Part print with two shaded views. Sizes in mm from the minimum x, y, z corner. A direction names the side the tool comes from. Give positions to 0.01 mm unless a question says otherwise; leave off trailing zeros. Write each loop counter-clockwise with the first axis right and the second up, starting at its lowest first coordinate (ties: lowest second). Pieces come first, ordered by that corner, then holes. Notation, with made-up numbers: (22, -18.5) -> (28, -18.5) arc R14 ccw to (28, -1.5) -> close; hole circle Ø3 at (-35, 38.5). An arc over 180 degrees is marked (long way). Write item = value, one per line. Start each with the question number.
Q1. Saw through at A-A, the plane y = 37.5. List the corners of the cut face in (x, z).
Q2. Mould opens along X. For the marked faces 1, 2, 3 and 4 say: pulls with the +X half, pulls with the -X half, needs draft (parallel to the pull), parting line crosses it, or undercut.
Q3. Saw through at D-D, the plane x = 33. List the corners of the cut face in (y, z).
Q4. Tool access for the marked faces 5, 6 and 7: list every direction of +Z, -Z, +X, -X, +Y, -Y with a clear straight run to the whole face (end or side of a thin tool).
Q5. Saw through at C-C, the plane y = 22. List the corners of the cut face in (x, z), then the cut area to 3 significant figures.
Q6. Drop flat-ended pins along their axis: P1, Ø1.2, axis at x = 62, z = 62.5, coming from the +Y side; P2, Ø6, axis at x = 54, z = 7.5, coming from the +Y side; P3, Ø4, axis at x = 30.5, z = 30.5, coming from the +Y side. Give the stop position or say it passes through.
Q7. Saw through at B-B, the plane z = 33. List the corners of the cut face in (x, y), then the cut area to 3 significant figures.
Q8. Wall check: line 1 (X direction, y = 36, z = 62); line 2 (Z direction, x = 62, y = 32); line 3 (X direction, y = 32, z = 33.5) (3 decimals). Give the ranges that are in metal, low to high.
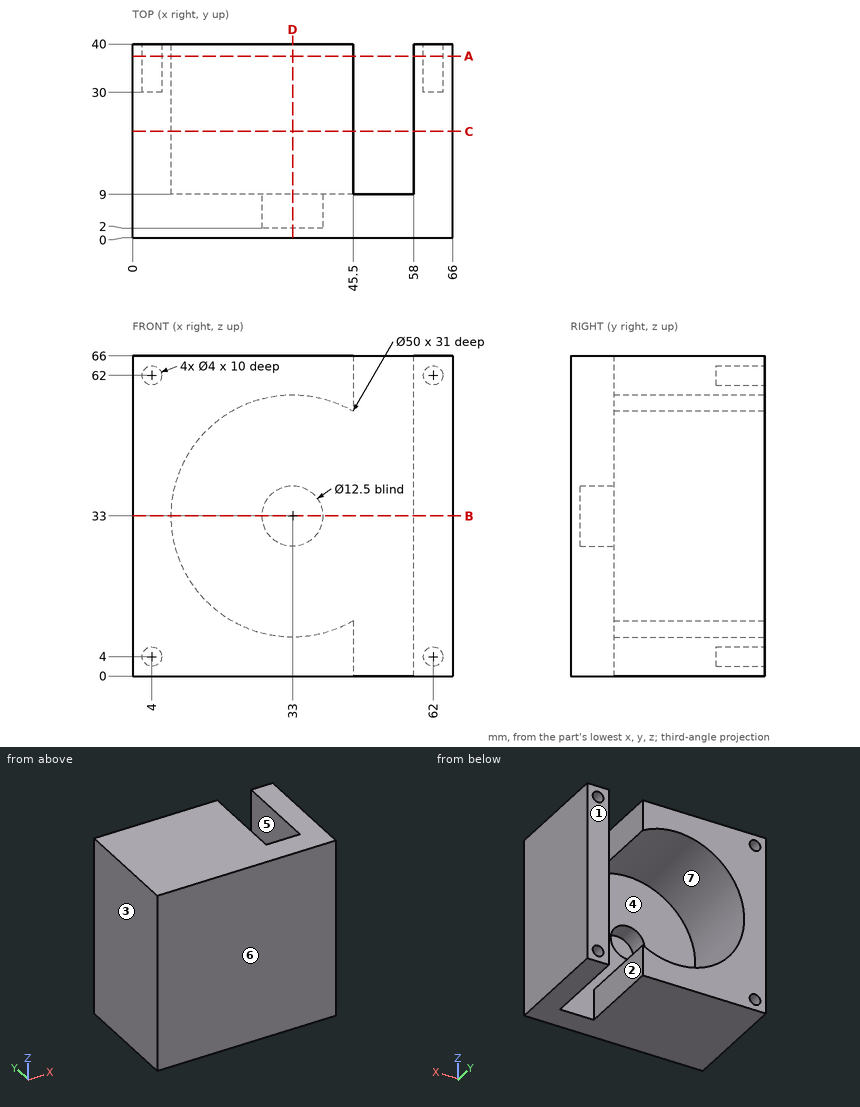
Report:
q1.outline = (0, 0) -> (45.5, 0) -> (45.5, 11.35) arc R25 cw (long way) to (45.5, 54.65) -> (45.5, 66) -> (0, 66) -> close; (58, 0) -> (66, 0) -> (66, 66) -> (58, 66) -> close; hole circle Ø4 at (4, 4); hole circle Ø4 at (4, 62); hole circle Ø4 at (62, 4); hole circle Ø4 at (62, 62)
q2.face_1 = needs draft
q2.face_2 = undercut
q2.face_3 = pulls with the -X half
q2.face_4 = undercut
q3.outline = (0, 0) -> (40, 0) -> (40, 8) -> (9, 8) -> (9, 26.75) -> (2, 26.75) -> (2, 39.25) -> (9, 39.25) -> (9, 58) -> (40, 58) -> (40, 66) -> (0, 66) -> close
q4.face_5 = +Z, -Z, +Y
q4.face_6 = +Z, -Z, +X, -X, -Y
q4.face_7 = +Y
q5.outline = (0, 0) -> (45.5, 0) -> (45.5, 11.35) arc R25 cw (long way) to (45.5, 54.65) -> (45.5, 66) -> (0, 66) -> close; (58, 0) -> (66, 0) -> (66, 66) -> (58, 66) -> close
q5.area = 1,950 mm2
q6.P1 = 30
q6.P2 = 9
q6.P3 = 2
q7.outline = (0, 0) -> (66, 0) -> (66, 40) -> (58, 40) -> (58, 9) -> (39.25, 9) -> (39.25, 2) -> (26.75, 2) -> (26.75, 9) -> (8, 9) -> (8, 40) -> (0, 40) -> close
q7.area = 1,000 mm2
q8.line_1 = 0 to 2, 6 to 45.5, 58 to 60, 64 to 66
q8.line_2 = 0 to 2, 6 to 60, 64 to 66
q8.line_3 = 0 to 8.005, 58 to 66
